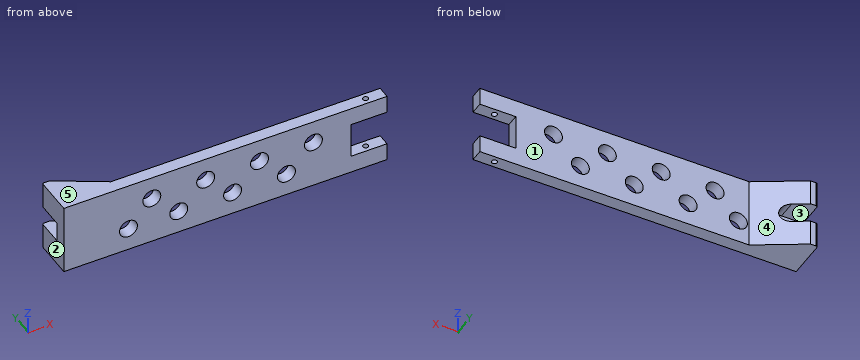
```python
from build123d import *

# Parameters (mm, degrees)
CYLINDER009_R          = 5
CYLINDER009_DEPTH      = 20
CYLINDER009_ROLL_ANGLE = 90
CYLINDER008_R          = 5
CYLINDER008_DEPTH      = 20
CYLINDER008_ROLL_ANGLE = 90
CYLINDER007_R          = 5
CYLINDER007_DEPTH      = 20
CYLINDER007_ROLL_ANGLE = 90
CYLINDER006_R          = 5
CYLINDER006_DEPTH      = 20
CYLINDER006_ROLL_ANGLE = 90
CYLINDER005_R          = 5
CYLINDER005_DEPTH      = 20
CYLINDER005_ROLL_ANGLE = 90
CYLINDER004_R          = 5
CYLINDER004_DEPTH      = 20
CYLINDER004_ROLL_ANGLE = 90
CYLINDER002_R          = 5
CYLINDER002_DEPTH      = 20
CYLINDER002_ROLL_ANGLE = 90
CYLINDER003_R          = 5
CYLINDER003_DEPTH      = 20
CYLINDER003_ROLL_ANGLE = 90
CYLINDER_R             = 1.5
CYLINDER_DEPTH         = 50
BOX003_W               = 20
BOX003_H               = 10
BOX003_DEPTH           = 20
BOX_W                  = 180
BOX_H                  = 7
BOX_DEPTH              = 40
BOX004_W               = 40
BOX004_H               = 20
BOX004_DEPTH           = 11
CYLINDER001_R          = 5.5
CYLINDER001_DEPTH      = 28
CYLINDER001_ROLL_ANGLE = 90
BOX002_W               = 30
BOX002_H               = 15
BOX002_DEPTH           = 40
BOX002_PLACEMENT_ANGLE = 30
BOX001_W               = 30
BOX001_H               = 15
BOX001_DEPTH           = 40
FILLET_R               = 1


with BuildPart() as cilindro008:
    # Cylinder009 → Cylinder009 (new body)
    with BuildSketch(Plane.XY):
        Circle(CYLINDER009_R)
    extrude(amount=CYLINDER009_DEPTH)


with BuildPart() as cilindro008_1:
    # Cylinder009 roll: moved
    add(cilindro008.part.rotate(Axis((0, 0, 0), (1, 0, 0)), CYLINDER009_ROLL_ANGLE))


with BuildPart() as cilindro008_2:
    # Cylinder009 placement: moved
    add(cilindro008_1.part.moved(Location((37, 15, 53))))


with BuildPart() as cilindro007:
    # Cylinder008 → Cylinder008 (new body)
    with BuildSketch(Plane.XY):
        Circle(CYLINDER008_R)
    extrude(amount=CYLINDER008_DEPTH)


with BuildPart() as cilindro007_1:
    # Cylinder008 roll: moved
    add(cilindro007.part.rotate(Axis((0, 0, 0), (1, 0, 0)), CYLINDER008_ROLL_ANGLE))


with BuildPart() as cilindro007_2:
    # Cylinder008 placement: moved
    add(cilindro007_1.part.moved(Location((50, 15, 67))))


with BuildPart() as cilindro006:
    # Cylinder007 → Cylinder007 (new body)
    with BuildSketch(Plane.XY):
        Circle(CYLINDER007_R)
    extrude(amount=CYLINDER007_DEPTH)


with BuildPart() as cilindro006_1:
    # Cylinder007 roll: moved
    add(cilindro006.part.rotate(Axis((0, 0, 0), (1, 0, 0)), CYLINDER007_ROLL_ANGLE))


with BuildPart() as cilindro006_2:
    # Cylinder007 placement: moved
    add(cilindro006_1.part.moved(Location((65, 15, 53))))


with BuildPart() as cilindro005:
    # Cylinder006 → Cylinder006 (new body)
    with BuildSketch(Plane.XY):
        Circle(CYLINDER006_R)
    extrude(amount=CYLINDER006_DEPTH)


with BuildPart() as cilindro005_1:
    # Cylinder006 roll: moved
    add(cilindro005.part.rotate(Axis((0, 0, 0), (1, 0, 0)), CYLINDER006_ROLL_ANGLE))


with BuildPart() as cilindro005_2:
    # Cylinder006 placement: moved
    add(cilindro005_1.part.moved(Location((80, 15, 67))))


with BuildPart() as cilindro004:
    # Cylinder005 → Cylinder005 (new body)
    with BuildSketch(Plane.XY):
        Circle(CYLINDER005_R)
    extrude(amount=CYLINDER005_DEPTH)


with BuildPart() as cilindro004_1:
    # Cylinder005 roll: moved
    add(cilindro004.part.rotate(Axis((0, 0, 0), (1, 0, 0)), CYLINDER005_ROLL_ANGLE))


with BuildPart() as cilindro004_2:
    # Cylinder005 placement: moved
    add(cilindro004_1.part.moved(Location((95, 15, 53))))


with BuildPart() as cilindro003:
    # Cylinder004 → Cylinder004 (new body)
    with BuildSketch(Plane.XY):
        Circle(CYLINDER004_R)
    extrude(amount=CYLINDER004_DEPTH)


with BuildPart() as cilindro003_1:
    # Cylinder004 roll: moved
    add(cilindro003.part.rotate(Axis((0, 0, 0), (1, 0, 0)), CYLINDER004_ROLL_ANGLE))


with BuildPart() as cilindro003_2:
    # Cylinder004 placement: moved
    add(cilindro003_1.part.moved(Location((110, 15, 67))))


with BuildPart() as cilindro001:
    # Cylinder002 → Cylinder002 (new body)
    with BuildSketch(Plane.XY):
        Circle(CYLINDER002_R)
    extrude(amount=CYLINDER002_DEPTH)


with BuildPart() as cilindro001_1:
    # Cylinder002 roll: moved
    add(cilindro001.part.rotate(Axis((0, 0, 0), (1, 0, 0)), CYLINDER002_ROLL_ANGLE))


with BuildPart() as cilindro001_2:
    # Cylinder002 placement: moved
    add(cilindro001_1.part.moved(Location((125, 15, 53))))


with BuildPart() as cilindro002:
    # Cylinder003 → Cylinder003 (new body)
    with BuildSketch(Plane.XY):
        Circle(CYLINDER003_R)
    extrude(amount=CYLINDER003_DEPTH)


with BuildPart() as cilindro002_1:
    # Cylinder003 roll: moved
    add(cilindro002.part.rotate(Axis((0, 0, 0), (1, 0, 0)), CYLINDER003_ROLL_ANGLE))


with BuildPart() as cilindro002_2:
    # Cylinder003 placement: moved
    add(cilindro002_1.part.moved(Location((140, 15, 67))))


with BuildPart() as agujero_tornillo:
    # Cylinder → Cylinder (new body)
    with BuildSketch(Plane(origin=(170, 3.5, 35), x_dir=(1, 0, 0), z_dir=(0, 0, 1))):
        Circle(CYLINDER_R)
    extrude(amount=CYLINDER_DEPTH)


with BuildPart() as cubo:
    # Box003 → Box003 (new body)
    with BuildSketch(Plane(origin=(160, 0, 50), x_dir=(1, 0, 0), z_dir=(0, 0, 1))):
        with Locations((10, 5)):
            Rectangle(BOX003_W, BOX003_H)
    extrude(amount=BOX003_DEPTH)


with BuildPart() as cut012:
    # Box → Box (new body)
    with BuildSketch(Plane.XY.offset(40)):
        with Locations((90, 3.5)):
            Rectangle(BOX_W, BOX_H)
    extrude(amount=BOX_DEPTH)

    # Cut001: cut Cubo
    add(cubo.part, mode=Mode.SUBTRACT)

    # Cut002: cut Agujero tornillo
    add(agujero_tornillo.part, mode=Mode.SUBTRACT)


with BuildPart() as cut012_1:
    # Cut002 placement: moved
    add(cut012.part.moved(Location((1, 0, 0))))

    # Cut005: cut Cilindro002
    add(cilindro002_2.part, mode=Mode.SUBTRACT)

    # Cut006: cut Cilindro001
    add(cilindro001_2.part, mode=Mode.SUBTRACT)

    # Cut007: cut Cilindro003
    add(cilindro003_2.part, mode=Mode.SUBTRACT)

    # Cut008: cut Cilindro004
    add(cilindro004_2.part, mode=Mode.SUBTRACT)

    # Cut009: cut Cilindro005
    add(cilindro005_2.part, mode=Mode.SUBTRACT)

    # Cut010: cut Cilindro006
    add(cilindro006_2.part, mode=Mode.SUBTRACT)

    # Cut011: cut Cilindro007
    add(cilindro007_2.part, mode=Mode.SUBTRACT)

    # Cut012: cut Cilindro008
    add(cilindro008_2.part, mode=Mode.SUBTRACT)


with BuildPart() as cubo001:
    # Box004 → Box004 (new body)
    with BuildSketch(Plane(origin=(-28, 7, 54.5), x_dir=(1, 0, 0), z_dir=(0, 0, 1))):
        with Locations((20, 10)):
            Rectangle(BOX004_W, BOX004_H)
    extrude(amount=BOX004_DEPTH)


with BuildPart() as cilindro:
    # Cylinder001 → Cylinder001 (new body)
    with BuildSketch(Plane.XY):
        Circle(CYLINDER001_R)
    extrude(amount=CYLINDER001_DEPTH)


with BuildPart() as cilindro_1:
    # Cylinder001 roll: moved
    add(cilindro.part.rotate(Axis((0, 0, 0), (1, 0, 0)), CYLINDER001_ROLL_ANGLE))


with BuildPart() as cilindro_2:
    # Cylinder001 placement: moved
    add(cilindro_1.part.moved(Location((12, 33, 60))))


with BuildPart() as cu_a001:
    # Box002 → Box002 (new body)
    with BuildSketch(Plane.XY):
        with Locations((15, 7.5)):
            Rectangle(BOX002_W, BOX002_H)
    extrude(amount=BOX002_DEPTH)


with BuildPart() as cu_a001_1:
    # Box002 placement: moved
    add(cu_a001.part.moved(Location((4, 22, 40))).rotate(Axis((4, 22, 40), (0, 0, -1)), BOX002_PLACEMENT_ANGLE))


with BuildPart() as fusion:
    # Box001 → Box001 (new body)
    with BuildSketch(Plane(origin=(0, 7, 40), x_dir=(1, 0, 0), z_dir=(0, 0, 1))):
        with Locations((15, 7.5)):
            Rectangle(BOX001_W, BOX001_H)
    extrude(amount=BOX001_DEPTH)

    add(cu_a001_1.part, mode=Mode.SUBTRACT)

    # Fillet
    fillet_edges = [fusion.edges().sort_by_distance(p)[0] for p in [
        (0, 22, 60),
    ]]
    fillet(fillet_edges, radius=FILLET_R)

    # Cut003: cut Cilindro
    add(cilindro_2.part, mode=Mode.SUBTRACT)

    # Cut004: cut Cubo001
    add(cubo001.part, mode=Mode.SUBTRACT)


with BuildPart() as fusion_1:
    # Cut004 placement: moved
    add(fusion.part.moved(Location((1, 0, 0))))

    # Fusion: union Cut012
    add(cut012_1.part)


solid = fusion_1.part
```
The listing builds one solid part. Answer for the finished solid, in the listing's coordinates (mm). Face numbers are marked on the shaded views. A direction names the side the tool comes from. Give positions to 0.01 mm unless a question says otherwise; leave off trailing zeros. Order: outer loops, then holes, each group sorted by start corner. A loop starts at its lowest first (then second) coordinate and runs counter-clockwise, first axis right, second up. Notation, with made-up numbers: (24.25, 10.5) -> (82.25, 10.5) arc R8 cw to (82.25, 25.5) -> close; hole circle Ø4 at (86.5, 31.5). An arc over 180 degrees is marked (long way). Answer as a JSON object with one key per item and string values. Group by question number.
Item 1: The part is cut by section C-C on x = 95. Write down the section's boundary in (y, z), and give its area (3 significant figures).
Item 2: Flat-ended cylindrical pins translate along their axes: pin 1 (6 mm diameter, centred on x = 140, z = 67, fed in from -Y); pin 2 (16 mm diameter, centred on x = 95, z = 53, fed in from +Y); pin 3 (13 mm diameter, centred on x = 37, z = 53, fed in from +Y); pin 4 (1.5 mm diameter, centred on y = 3, z = 60.5, fed in from +X). Find the tip coordinate at first contact, or state that the pin passes through.
Item 3: A tool of negligible diameter and unlimited length cuts with its end or side. For the marked faces 1 and 2, from which of +Z, -Z, +X, -X, +Y, -Y can it reach the whole face along a straight path? Write none if from no direction.
Item 4: Consider L1, parallel to X at y = 2.5, z = 53; L2, parallel to X at y = 4.75, z = 67; L3, parallel to X at y = 3.5, z = 72.5. Determine where each line is inside the solid, lowest interval first. Write a range as from..to.
Item 5: The part is cut by section A-A on y = 3.5. Give the number of separate pieces and of enclosed holes in the cut face, and give its area (3 significant figures).
Item 6: Determine the mould class of the marked faces 3, 4 and 5 for opening direction Z: pulls with the +Z half, pulls with the -Z half, needs draft (parallel to the pull), parting line crosses it, or undercut.
Item 7: The part is cut by section B-B on x = 171. Write down the section's boundary in (y, z).
Result set:
{
 "1": {"outline": "(0, 40) -> (7, 40) -> (7, 48) -> (0, 48) -> close; (0, 58) -> (7, 58) -> (7, 80) -> (0, 80) -> close", "area": "210 mm²"},
 "2": {"pin 1": "through", "pin 2": "y = 7", "pin 3": "y = 7.28", "pin 4": "x = 161"},
 "3": {"face 1": "+Z, -Z, +X, +Y", "face 2": "+Z, -Z, -X, +Y, -Y"},
 "4": {"L1": "1..32, 42..60, 70..90, 100..120, 130..161", "L2": "1..45, 55..75, 85..105, 115..135, 145..161", "L3": "1..169.5, 172.5..181"},
 "5": {"separate pieces": "3", "enclosed holes": "8", "area": "6,110 mm²"},
 "6": {"face 3": "undercut", "face 4": "needs draft", "face 5": "pulls with the +Z half"},
 "7": {"outline": "(0, 40) -> (2, 40) -> (2, 50) -> (0, 50) -> close; (0, 70) -> (2, 70) -> (2, 80) -> (0, 80) -> close; (5, 40) -> (7, 40) -> (7, 50) -> (5, 50) -> close; (5, 70) -> (7, 70) -> (7, 80) -> (5, 80) -> close"}
}
